The model under review builds one solid part; all positions refer to its coordinate system, in mm. A direction names the side the tool comes from. Coordinates: 2 decimals unless noted, no trailing zeros. Order: outer loops, then holes, each group sorted by start corner. A loop starts at its lowest first (then second) coordinate and runs counter-clockwise, first axis right, second up. Notation, with made-up numbers: (23.25, 0) -> (32.25, 0) arc R10 ccw to (32.25, 12) -> close; hole circle Ø8 at (27, -5). An arc over 180 degrees is marked (long way). Use one line per item in the form item = value.
from build123d import *

# Parameters (mm, degrees)
BOSS_EXTRUDE1_DEPTH   = 2
BOSS_EXTRUDE1_2_DEPTH = 2
BASE_W                = 20
BASE_H                = 70
BOSS_EXTRUDE2_DEPTH   = 2
SKETCH10_W            = 50
SKETCH10_H            = 30
BOSS_EXTRUDE3_DEPTH   = 2
SKETCH9_W             = 50
SKETCH9_H             = 30
BOSS_EXTRUDE4_DEPTH   = 2
SKETCH11_W            = 40
SKETCH11_H            = 5
BOSS_EXTRUDE5_DEPTH   = 2


with BuildPart() as part:
    # hook → Boss-Extrude1 (new body)
    with BuildSketch(Plane.XY):
        with BuildLine():
            Line((-10, 35), (-10, 25))
            Line((-10, 25), (-58.535533906, 73.535533906))
            ThreePointArc((-58.535533906, 73.535533906), (-59.619397663, 75.15765065), (-60, 77.071067812))
            Line((-60, 77.071067812), (-60, 85))
            ThreePointArc((-60, 85), (-58.535533906, 88.535533906), (-55, 90))
            Line((-55, 90), (-27.5, 90))
            ThreePointArc((-27.5, 90), (-25.732233047, 89.267766953), (-25, 87.5))
            Line((-25, 87.5), (-24.999999999, 76.499999999))
            ThreePointArc((-24.999999999, 76.499999999), (-25.439339828, 75.439339828), (-26.499999999, 74.999999999))
            Line((-26.499999999, 74.999999999), (-28.499999999, 74.999999999))
            ThreePointArc((-28.499999999, 74.999999999), (-29.560660171, 75.439339828), (-29.999999999, 76.499999999))
            Line((-29.999999999, 76.499999999), (-29.999999999, 84.999999999))
            Line((-29.999999999, 84.999999999), (-49.999999999, 84.999999999))
            Line((-49.999999999, 84.999999999), (-50, 77.071067812))
            ThreePointArc((-50, 77.071067812), (-49.619397663, 75.15765065), (-48.535533906, 73.535533906))
            Line((-48.535533906, 73.535533906), (-10, 35))
        make_face()
    extrude(amount=-BOSS_EXTRUDE1_DEPTH)



with BuildPart() as body_2:
    # hook → Boss-Extrude1 2 (new body)
    with BuildSketch(Plane.XY):
        with BuildLine():
            Line((48.535533906, 73.535533906), (10, 35))
            Line((10, 35), (10, 25))
            Line((10, 25), (58.535533906, 73.535533906))
            ThreePointArc((58.535533906, 73.535533906), (59.619397663, 75.15765065), (60, 77.071067812))
            Line((60, 77.071067812), (60, 85))
            ThreePointArc((60, 85), (58.535533906, 88.535533906), (55, 90))
            Line((55, 90), (27.5, 90))
            ThreePointArc((27.5, 90), (25.732233047, 89.267766953), (25, 87.5))
            Line((25, 87.5), (24.999999999, 76.499999999))
            ThreePointArc((24.999999999, 76.499999999), (25.439339828, 75.439339828), (26.499999999, 74.999999999))
            Line((26.499999999, 74.999999999), (28.499999999, 74.999999999))
            ThreePointArc((28.499999999, 74.999999999), (29.560660171, 75.439339828), (29.999999999, 76.499999999))
            Line((29.999999999, 76.499999999), (29.999999999, 84.999999999))
            Line((29.999999999, 84.999999999), (49.999999999, 84.999999999))
            Line((49.999999999, 84.999999999), (50, 77.071067812))
            ThreePointArc((50, 77.071067812), (49.619397663, 75.15765065), (48.535533906, 73.535533906))
        make_face()
    extrude(amount=-BOSS_EXTRUDE1_2_DEPTH)


with BuildPart() as part_1:
    add(part.part)

    add(body_2.part)  # Boss-Extrude2 merges body 2
    # base → Boss-Extrude2 (add)
    with BuildSketch(Plane.XY):
        Rectangle(BASE_W, BASE_H)
    extrude(amount=-BOSS_EXTRUDE2_DEPTH)

    # Sketch9 → Boss-Extrude4 (add)
    with BuildSketch(Plane(origin=(0, 35, 0), x_dir=(1, 0, 0), z_dir=(0, 1, 0))):
        with Locations((15, -15)):
            Rectangle(SKETCH9_W, SKETCH9_H)
    extrude(amount=-BOSS_EXTRUDE4_DEPTH)



with BuildPart() as body_2_2:
    # Sketch10 → Boss-Extrude3 (new body)
    with BuildSketch(Plane(origin=(0, -35, 0), x_dir=(1, 0, 0), z_dir=(0, 1, 0))):
        with Locations((15, -15)):
            Rectangle(SKETCH10_W, SKETCH10_H)
    extrude(amount=BOSS_EXTRUDE3_DEPTH)


with BuildPart() as part_2:
    add(part_1.part)

    add(body_2_2.part)  # Boss-Extrude5 merges body 2 2
    # Sketch11 → Boss-Extrude5 (add)
    with BuildSketch(Plane.XY.offset(30)):
        with Locations((10, -30.5)):
            Rectangle(SKETCH11_W, SKETCH11_H)
        with Locations((10, 30.5)):
            Rectangle(SKETCH11_W, SKETCH11_H)
    extrude(amount=-BOSS_EXTRUDE5_DEPTH)


solid = part_2.part
Item 1: We need section D-D (y = -2.5). Write out the cut boundary in (x, z).
Results found:
outline = (-10, -2) -> (10, -2) -> (10, 0) -> (-10, 0) -> close
Item 2: We need section A-A (x = -46). Write out the cut boundary in (y, z).
Results found:
outline = (61, -2) -> (71, -2) -> (71, 0) -> (61, 0) -> close; (85, -2) -> (90, -2) -> (90, 0) -> (85, 0) -> close
Item 3: We need section B-B (z = 25). Write out the cut boundary in (x, y).
Results found:
outline = (-10, -35) -> (40, -35) -> (40, -33) -> (-10, -33) -> close; (-10, 33) -> (40, 33) -> (40, 35) -> (-10, 35) -> close
Item 4: Tool access review of faces 5 (the face through (-30, 55, -1)), 6 (the face through (-10, 34, 19)), 7 (the face through (10, -30, 28)), 8 (the face through (42.3, 66.7, 0)): name each direction out of +Z, -Z, +X, -X, +Y, -Y from which nothing blocks a thin tool from reaching the whole face with its end or side.
Results found:
face_5 = +Z, -Z
face_6 = +Z, -X, +Y, -Y
face_7 = +X, -X
face_8 = +Z, +X, -X, +Y
Item 5: Draft analysis for pull direction X (two halves, no side actions). For faces 1 (the face through (59, 88, -1)), 2 (the face through (-10, -14, -1)), 3 (the face through (30, 55, -1)), 4 (the face through (9, 32, 30)), state which applies: released by +X, released by -X, zero draft, split by the parting line, or undercut.
Results found:
face_1 = released by +X
face_2 = released by -X
face_3 = undercut
face_4 = zero draft
Item 6: We need section C-C (x = 0). Write out the cut boundary in (y, z), plus the area to 3 significant figures.
Results found:
outline = (-35, -2) -> (35, -2) -> (35, 30) -> (28, 30) -> (28, 28) -> (33, 28) -> (33, 0) -> (-33, 0) -> (-33, 28) -> (-28, 28) -> (-28, 30) -> (-35, 30) -> close
area = 280 mm²
Item 7: Clearance check with flat-ended pins moving along their axes: pin 1 (0.6 mm diameter, centred on y = -29.5, z = 29, fed in from +X); pin 2 (1 mm diameter, centred on x = 3, z = 29, fed in from +Y); pin 3 (0.6 mm diameter, centred on x = 37, z = -1, fed in from -Y). State where each tip first meets the part, or that it passes through.
Results found:
pin_1 = 30
pin_2 = 35
pin_3 = 51.7
Item 8: To check wall thickness, follow L1, parallel to Y at x = 38, z = 24.5; L2, parallel to Z at x = 31.5, y = 85.5. State the ranges of each line that lie inside material, in increasing order. Write a range as from..to.
Results found:
L1 = -35..-33, 33..35
L2 = -2..0
